Source: CAD feature listing. Evaluate the final solid. Frame: model axes, mm. Round coordinates to 2 decimals unless told otherwise and drop trailing zeros. Order: outer loops, then holes, each group sorted by start corner. A loop starts at its lowest first (then second) coordinate and runs counter-clockwise, first axis right, second up. Notation, with made-up numbers: (-26.75, 53) -> (1.25, 53) arc R6 cw to (1.25, 58) -> close; hole circle Ø2 at (-21.75, -25). An arc over 180 degrees is marked (long way). Answer as CSV lines item,"result". Start each with the question number.
(1) Section query B-B (x = -44.37). Output: boundary loops of the cut face in (y, z).
(2) Section query A-A (y = 24.85). Output: boundary loops of the cut face in (x, z).
(3) Pull-direction query (Y, two-part tool) for faces 1 (the flat face through (1, 32.6, 1)), 2 (the flat face through (55.8, 0, 1)), 3 (the cylindrical face through (33.19, 25.88, 1.01)); classes: +Y half, -Y half, draft (parallel to the pull), parting line (faces both ways), or undercut.
(4) Contact query for a flat-ended pin moving along its axis: P1, Ø10, axis at x = 8.5, y = 20.5, coming from the -Z side. Output: stop coordinate, or through.
(5) Line query: line 1 along X through (y, z) = (24.85, 0.9); line 2 along Y through (x, z) = (31.84, 0.6); line 3 along Y through (x, z) = (-44.37, 1.35). Output: solid intervals per line, ascending. Write a range as from..to.
```python
from build123d import *

# Parameters (mm, degrees)
F1_DEPTH = 2
F2_D     = 3.4


with BuildPart() as f1:
    # F0 (on Top) → F1 (new body)
    with BuildSketch(Plane.XY):
        with BuildLine():
            Line((-54.8, -32.6), (54.8, -32.6))
            ThreePointArc((54.8, -32.6), (55.5071067812, -32.3071067812), (55.8, -31.6))
            Line((55.8, -31.6), (55.8, 31.6))
            ThreePointArc((55.8, 31.6), (55.5071067812, 32.3071067812), (54.8, 32.6))
            Line((54.8, 32.6), (-54.8, 32.6))
            ThreePointArc((-54.8, 32.6), (-55.5071067812, 32.3071067812), (-55.8, 31.6))
            Line((-55.8, 31.6), (-55.8, -31.6))
            ThreePointArc((-55.8, -31.6), (-55.5071067812, -32.3071067812), (-54.8, -32.6))
        make_face()
    extrude(amount=F1_DEPTH)

    # F2 (through all)
    with Locations(Plane(origin=(0, 0, 0), x_dir=(1, 0, 0), z_dir=(0, 0, -1))):
        with Locations((-50.71, -24.85), (-44.37, 23.41), (31.84, -24.85)):
            Hole(F2_D / 2)


solid = f1.part
```
Answer block:
1,outline,"(-32.6, 0) -> (-25.11, 0) -> (-25.11, 2) -> (-32.6, 2) -> close; (-21.71, 0) -> (32.6, 0) -> (32.6, 2) -> (-21.71, 2) -> close"
2,outline,"(-55.8, 0) -> (-52.41, 0) -> (-52.41, 2) -> (-55.8, 2) -> close; (-49.01, 0) -> (30.14, 0) -> (30.14, 2) -> (-49.01, 2) -> close; (33.54, 0) -> (55.8, 0) -> (55.8, 2) -> (33.54, 2) -> close"
3,face 1,"+Y half"
3,face 2,"draft"
3,face 3,"undercut"
4,P1,"z = 0"
5,line 1,"-55.8..-52.41, -49.01..30.14, 33.54..55.8"
5,line 2,"-32.6..23.15, 26.55..32.6"
5,line 3,"-32.6..-25.11, -21.71..32.6"
